Geometry: final body of the model. Coordinates: model frame, mm. A direction names the side the tool comes from. Give positions to 0.01 mm unless a question says otherwise; leave off trailing zeros. Order: outer loops, then holes, each group sorted by start corner. A loop starts at its lowest first (then second) coordinate and runs counter-clockwise, first axis right, second up. Notation, with made-up numbers: M 65,-18.75 L 97,-18.75 A12 cw 97,0.25 Z; hole C 54.25,49 d2. An arc over 180 degrees is marked long. Use CSV: the item, a comma, the result in double quotes.
Autodesk Inventor part; units mm, degrees
ref_plane "YZ Plane" through (0, 0, 0) normal (1, 0, 0) x (0, 1, 0)
ref_plane "XZ Plane" through (0, 0, 0) normal (0, 1, 0) x (-1, 0, 0)
ref_plane "XY Plane" through (0, 0, 0) normal (0, 0, 1) x (1, 0, 0)
sketch "Sketch1" plane through (0, 0, 0) normal (0, 0, 1) x (1, 0, 0)
  line L0 (0, 0) -> (31.75, 0)
  line L1 (31.75, 0) -> (31.75, 25.4)
  line L2 (31.75, 25.4) -> (19.05, 25.4)
  line L3 (19.05, 25.4) -> (19.05, 12.7)
  line L4 (19.05, 12.7) -> (0, 12.7)
  line L5 (0, 12.7) -> (0, 0)
  dimension "d0" = 31.75
  dimension "d1" = 25.4
  dimension "d2" = 12.7
  dimension "d3" = 12.7
extrude "Extrusion1" add sketch "Sketch1" along normal blind 19.05
fillet "Fillet1" radius 3.175 3 edges at (0, 6.35, 19.05) (19.05, 12.7, 9.525) (0, 6.35, 0)
sketch "Sketch2" plane through (3.175, 12.7, 0) normal (0, 1, 0) x (1, 0, 0)
  line L0 (15.875, 0) -> (12.7, 0)
  circle A0 centre (6.35, -9.4797) radius 4.7625
  point P0 (-3.175, 0)
  dimension "d7" = 9.525
extrude "Extrusion2" cut sketch "Sketch2" against normal blind 12.7
mirror "Mirror1" about plane through (31.75, 0, 0) normal (1, 0, 0) of "Extrusion1", "Extrusion2", "Fillet1"
properties part number "Mirror 3D"
1. Pin query (flat end, axial travel): pin 1 Ø4 at (x, y) = (11.5, 11.5) entering from -Z; pin 2 Ø3 at (y, z) = (16.5, 17) entering from -X; pin 3 Ø7.5 at (x, z) = (53.98, 9.48) entering from +Y; pin 4 Ø3 at (y, z) = (21.5, 12) entering from +X. Return the tip coordinate at first contact, or that it passes through.
Answer:
pin 1,"z = 0"
pin 2,"x = 18.93"
pin 3,"through"
pin 4,"x = 44.45"
2. Section B-B, the plane y = 2. Give the number of separate pieces and of enclosed holes in the cut face, plus the area to 3 significant figures.
Answer:
separate pieces,"1"
enclosed holes,"2"
area,"1,060 mm2"
3. Line query: line 1 (X direction, y = 5.75, z = 9); line 2 (X direction, y = 3.25, z = 7.75); line 3 (Y direction, x = 5.5, z = 16.75). Output: solid intervals per line, ascending.
Answer:
line 1,"0 to 4.79, 14.26 to 49.24, 58.71 to 63.5"
line 2,"0 to 5.09, 13.96 to 49.54, 58.41 to 63.5"
line 3,"0 to 12.7"
4. Reachability of faces 1 (the face through (44.45, 21, 9)), 2 (the face through (63.5, 6, 9)), 3 (the face through (4.5, 12.7, 9.4)) from +Z, -Z, +X, -X, +Y, -Y: full face, straight path, thin tool, end or side. Return the list, or none.
Answer:
face 1,"+Z, -Z, +X, +Y"
face 2,"+Z, -Z, +X, +Y, -Y"
face 3,"+Z, -Z, -X, +Y"
5. Section A-A, the plane z = 3.75. Return the cut outline in (x, y) (3 decimals), plus the area to 3 significant figures.
Answer:
outline,"M 0,0 L 63.5,0 L 63.5,12.7 L 47.625,12.7 A3.175 cw 44.45,15.875 L 44.45,25.4 L 19.05,25.4 L 19.05,15.875 A3.175 cw 15.875,12.7 L 0,12.7 Z"
area,"1,130 mm2"
6. Pull-direction query (X, two-part tool) for faces 4 (the face through (62.55, 6.26, 0.91)), 5 (the face through (58.733, 6.439, 9.689)), 6 (the face through (31, 10, 19.05)); classes: +X half, -X half, draft (parallel to the pull), parting line (faces both ways), or undercut.
Answer:
face 4,"+X half"
face 5,"undercut"
face 6,"draft"
7. Section C-C, the plane x = 7.5. Return the cut outline in (y, z).
Answer:
outline,"M 0,0 L 12.7,0 L 12.7,5.17 L 0,5.17 Z; M 0,13.79 L 12.7,13.79 L 12.7,19.05 L 0,19.05 Z"
8. Section D-D, the plane z = 7.5. Return the cut outline in (x, y) (3 decimals), plus the area to 3 significant figures.
Answer:
outline,"M 0,0 L 5.193,0 L 5.193,12.7 L 0,12.7 Z; M 13.857,0 L 49.643,0 L 49.643,12.7 L 47.625,12.7 A3.175 cw 44.45,15.875 L 44.45,25.4 L 19.05,25.4 L 19.05,15.875 A3.175 cw 15.875,12.7 L 13.857,12.7 Z; M 58.307,0 L 63.5,0 L 63.5,12.7 L 58.307,12.7 Z"
area,"913 mm2"
